```python
from build123d import *

# Parameters (mm, degrees)
SKETCH_1_W          = 91
SKETCH_1_H          = 44
EXTRUDE_1_DEPTH     = 1.5
SKETCH_2_W          = 61
SKETCH_2_H          = 43
EXTRUDE_2_DEPTH     = 2.5
SKETCH_3_R          = 1.75
CUT_EXTRUDE_1_DEPTH = 2.5
SKETCH_4_W          = 12
SKETCH_4_H          = 12
EXTRUDE_3_DEPTH     = 6.7
SKETCH_5_W          = 12
SKETCH_5_H          = 12
CUT_EXTRUDE_2_DEPTH = 3.4
SKETCH_6_R          = 1
EXTRUDE_4_DEPTH     = 2
SKETCH_7_R          = 7
EXTRUDE_5_DEPTH     = 14
SKETCH_8_R          = 3.25
EXTRUDE_6_DEPTH     = 8


with BuildPart() as part:
    # 草图1 → 凸台-拉伸1 (new body)
    with BuildSketch(Plane(origin=(0, 0, 0), x_dir=(1, 0, 0), z_dir=(0, 1, 0))):
        with Locations((45.5, 22)):
            Rectangle(SKETCH_1_W, SKETCH_1_H)
    extrude(amount=EXTRUDE_1_DEPTH)

    # 草图2 → 凸台-拉伸2 (add)
    with BuildSketch(Plane(origin=(0, 1.5, 0), x_dir=(1, 0, 0), z_dir=(0, 1, 0))):
        with Locations((36.5, 22)):
            Rectangle(SKETCH_2_W, SKETCH_2_H)
    extrude(amount=EXTRUDE_2_DEPTH)

    # 草图3 → 切除-拉伸1 (cut)
    with BuildSketch(Plane(origin=(0, 1.5, 0), x_dir=(1, 0, 0), z_dir=(0, 1, 0))):
        with Locations(Location((87.65, 40.75, 0), (0, 0, 270))):
            Circle(SKETCH_3_R)
        with Locations(Location((87.65, 3.25, 0), (0, 0, 270))):
            Circle(SKETCH_3_R)
        with Locations(Location((3.15, 3.25, 0), (0, 0, 270))):
            Circle(SKETCH_3_R)
        with Locations(Location((3.15, 40.75, 0), (0, 0, 270))):
            Circle(SKETCH_3_R)
    extrude(amount=-CUT_EXTRUDE_1_DEPTH, mode=Mode.SUBTRACT)

    # 草图4 → 凸台-拉伸3 (add)
    with BuildSketch(Plane(origin=(0, 1.5, 0), x_dir=(1, 0, 0), z_dir=(0, 1, 0))):
        with Locations((79, 31.4)):
            Rectangle(SKETCH_4_W, SKETCH_4_H)
        with Locations((79, 13)):
            Rectangle(SKETCH_4_W, SKETCH_4_H)
    extrude(amount=EXTRUDE_3_DEPTH)

    # 草图5 → 切除-拉伸2 (cut)
    with BuildSketch(Plane(origin=(0, 8.2, 0), x_dir=(1, 0, 0), z_dir=(0, 1, 0))):
        with Locations((79, 13)):
            Rectangle(SKETCH_5_W, SKETCH_5_H)
    extrude(amount=-CUT_EXTRUDE_2_DEPTH, mode=Mode.SUBTRACT)

    # 草图6 → 凸台-拉伸4 (add)
    with BuildSketch(Plane(origin=(0, 8.2, 0), x_dir=(1, 0, 0), z_dir=(0, 1, 0))):
        with Locations(Location((79, 31.4, 0), (0, 0, 270))):
            Circle(SKETCH_6_R)
    extrude(amount=EXTRUDE_4_DEPTH)

    # 草图7 → 凸台-拉伸5 (add)
    with BuildSketch(Plane(origin=(0, 10.2, 0), x_dir=(1, 0, 0), z_dir=(0, 1, 0))):
        with Locations(Location((79, 31.4, 0), (0, 0, 270))):
            Circle(SKETCH_7_R)
    extrude(amount=EXTRUDE_5_DEPTH)

    # 草图8 → 凸台-拉伸6 (add)
    with BuildSketch(Plane(origin=(0, 4.8, 0), x_dir=(1, 0, 0), z_dir=(0, 1, 0))):
        with Locations(Location((79, 13, 0), (0, 0, 270))):
            Circle(SKETCH_8_R)
    extrude(amount=EXTRUDE_6_DEPTH)


solid = part.part
```
The listing builds one solid part. Answer for the finished solid, in the listing's coordinates (mm). A direction names the side the tool comes from. Round coordinates to 2 decimals unless told otherwise and drop trailing zeros. Order: outer loops, then holes, each group sorted by start corner. A loop starts at its lowest first (then second) coordinate and runs counter-clockwise, first axis right, second up. Notation, with made-up numbers: (68, 41) - (114, 41) arc R19 cw to (114, 74) - close; hole circle Ø7 at (83.5, 65.25). An arc over 180 degrees is marked (long way). Put each result on its own line as item: value. Start each with the question number.
(1) Given P1, Ø21.5, axis at x = 31, z = -16, coming from the +Y side; P2, Ø9.5, axis at x = 78.5, z = -12.5, coming from the +Y side; P3, Ø3, axis at x = 70.5, z = -14.5, coming from the +Y side, each flat-ended and moving along its own axis, determine where each tip first touches the part or whether it passes through.
(2) Find section A-A (z = -40.75). Give the vertices of the cut face in (x, y).
(3) Determine the mould class of faces 6 (the flat face through (73, 5, -31)), 7 (the flat face through (79, 5, -37.4)), 8 (the cylindrical face through (78.4, 9.2, -32.2)) for opening direction Z: released by +Z, released by -Z, zero draft, split by the parting line, or undercut.
(4) For faces 1 (the flat face through (36, 3, -0.5)), 2 (the flat face through (36, 4, -22)), 3 (the flat face through (67, 3, -22)), 4 (the flat face through (36, 3, -43.5)), 5 (the cylindrical face through (85.94, 17.1, -32.31)), determine the directions among +Z, -Z, +X, -X, +Y, -Y from which every point of the face is accessible in a straight line to the end or side of a thin tool.
(5) Find section C-C (z = -13). Give the vertices of the cut face in (x, y), plus the area to 3 significant figures.
(6) Find section B-B (x = 3.15). Give the vertices of the cut face in (y, z).
(7) Straight lines are drawn through the part: probe 1 along Z at (x, y) = (87.65, 0.75); probe 2 along X at (y, z) = (2.25, -17); probe 3 along Y at (x, z) = (37.5, -8.5). For each, find the intervals that lie inside material, in ascending order. Write a range as from..to.
(8) Find section D-D (x = 79). Give the vertices of the cut face in (y, z), plus the area to 3 significant figures.
Reply:
1. P1: y = 4
1. P2: y = 12.8
1. P3: y = 1.5
2. outline: (0, 0) - (1.4, 0) - (1.4, 1.5) - (0, 1.5) - close; (4.9, 0) - (85.9, 0) - (85.9, 1.5) - (67, 1.5) - (67, 4) - (6, 4) - (6, 1.5) - (4.9, 1.5) - close; (89.4, 0) - (91, 0) - (91, 1.5) - (89.4, 1.5) - close
3. face 6: zero draft
3. face 7: released by -Z
3. face 8: undercut
4. face 1: +Z, +X, -X, +Y
4. face 2: +Z, -Z, -X, +Y
4. face 3: +Z, -Z, +Y
4. face 4: -Z, +X, -X, +Y
4. face 5: +Y
5. outline: (0, 0) - (91, 0) - (91, 1.5) - (85, 1.5) - (85, 4.8) - (82.25, 4.8) - (82.25, 12.8) - (75.75, 12.8) - (75.75, 4.8) - (73, 4.8) - (73, 1.5) - (67, 1.5) - (67, 4) - (6, 4) - (6, 1.5) - (0, 1.5) - close
5. area: 381 mm^2
6. outline: (0, -44) - (1.5, -44) - (1.5, -42.5) - (0, -42.5) - close; (0, -39) - (1.5, -39) - (1.5, -5) - (0, -5) - close; (0, -1.5) - (1.5, -1.5) - (1.5, 0) - (0, 0) - close
7. probe 1: -44..-42.5, -39..-5, -1.5..0
7. probe 2: 6..67, 73..85
7. probe 3: 0..4
8. outline: (0, -44) - (1.5, -44) - (1.5, -37.4) - (8.2, -37.4) - (8.2, -32.4) - (10.2, -32.4) - (10.2, -38.4) - (24.2, -38.4) - (24.2, -24.4) - (10.2, -24.4) - (10.2, -30.4) - (8.2, -30.4) - (8.2, -25.4) - (1.5, -25.4) - (1.5, -19) - (4.8, -19) - (4.8, -16.25) - (12.8, -16.25) - (12.8, -9.75) - (4.8, -9.75) - (4.8, -7) - (1.5, -7) - (1.5, 0) - (0, 0) - close
8. area: 438 mm^2
